Source: CAD feature listing. Evaluate the final solid. Frame: model axes, mm. Face numbers are marked on the shaded views. Give positions to 0.01 mm unless a question says otherwise; leave off trailing zeros. Order: outer loops, then holes, each group sorted by start corner. A loop starts at its lowest first (then second) coordinate and runs counter-clockwise, first axis right, second up.
1) First-contact query: P1, Ø6.5, axis at x = 42, y = 47.5, coming from the -Z side; P2, Ø10, axis at x = 44.5, z = 15.5, coming from the +Y side; P3, Ø2, axis at y = 30.5, z = 9, coming from the +X side; P4, Ø14.5, axis at y = 16, z = 44, coming from the -X side. Flat tips, straight axial feed; report the tip coordinate or a pass-through.
2) Section B-B, the plane z = 27. Return loops of the section in (x, y).
3) Material intervals for line 1 (X direction, y = 20, z = 32.5); line 2 (Z direction, x = 16.5, y = 19); line 3 (Y direction, x = 1.1, z = 44), sorted ascending.
4) Section A-A, the plane x = 12.5. Return loops of the section in (y, z).
5) Section C-C, the plane y = 9.5. Return loops of the section in (x, z).
6) Draft query along X for the marked faces 1, 2, 3 and 4. Return one class per face: released by +X, released by -X, zero draft, split by the parting line, or undercut.
7) Section D-D, the plane z = 7. Return loops of the section in (x, y).
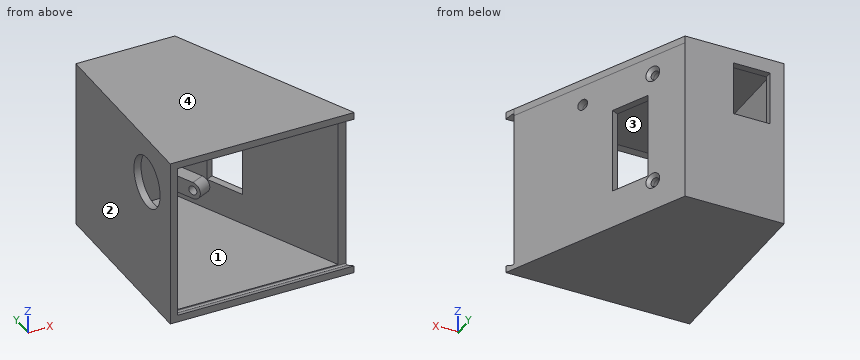
Autodesk Inventor part; units mm, degrees
ref_plane "Work Plane1" through (65, 0, 57.5) normal (1, 0, 0) x (0, 0, -1)
ref_plane "YZ Plane" through (0, 0, 0) normal (1, 0, 0) x (0, 1, 0)
ref_plane "XZ Plane" through (0, 0, 0) normal (0, 1, 0) x (-1, 0, 0)
sketch "Sketch1" plane through (0, 0, 0) normal (0, 0, 1) x (1, 0, 0)
  line L0 (0, 0) -> (0, 65)
  line L1 (0, 65) -> (35, 65)
  line L2 (35, 65) -> (65, 0)
  line L3 (65, 0) -> (0, 0)
  line L4 (35, 65) -> (19.5647, 57.876) construction
  line L5 (19.5647, 57.876) -> (40.0985, 13.386) construction
  line L6 (40.0985, 13.386) -> (55.5339, 20.51) construction
  line L7 (5, 65) -> (5, 39) construction
  line L8 (5, 39) -> (17.8, 39) construction
  line L9 (17.8, 39) -> (17.8, 65) construction
  line L10 (0, 23.6) -> (40, 23.6) construction
  line L11 (40, 23.6) -> (40, 6) construction
  line L12 (40, 6) -> (0, 6) construction
  line L13 (0, 26.5) -> (11, 26.5) construction
  line L14 (11, 26.5) -> (11, 23.6) construction
  line L15 (11, 6) -> (11, 3.1) construction
  line L16 (11, 3.1) -> (0, 3.1) construction
  dimension "d27" = 17
  dimension "d28" = 12.8
  dimension "d29" = 5
  dimension "d31" = 40
  dimension "d32" = 17.6
  dimension "d33" = 26
  dimension "d34" = 35
  dimension "d35" = 65
  dimension "d36" = 23.4
  dimension "d37" = 11
  dimension "d38" = 49
  dimension "d39" = 65
  dimension "d40" = 6
extrude "Extrusion1" add sketch "Sketch1" along normal blind 2.5
sketch "Sketch2" plane through (0, 0, 2.5) normal (0, 0, 1) x (1, 0, 0)
  line L0 (0, 65) -> (0, 0)
  line L1 (0, 0) -> (65, 0)
  line L2 (65, 0) -> (35, 65)
  line L3 (35, 65) -> (0, 65)
  line L4 (2.5, 2.5) -> (2.5, 62.5)
  line L5 (2.5, 62.5) -> (33.4004, 62.5)
  line L6 (33.4004, 62.5) -> (61.0927, 2.5)
  line L7 (61.0927, 2.5) -> (2.5, 2.5)
  line L8 (2.5, 2.5) -> (2.5, 0)
  line L9 (60.862, 3) -> (63.6154, 3)
  dimension "d2" = 2.5
  dimension "d3" = 3
extrude "Extrusion2" add sketch "Sketch2" along normal blind 55 contours L3 L2 L9 L6 L5 L4 L8 L1 L0
sketch "Sketch3" plane through (0, 0, 57.5) normal (0, 0, 1) x (1, 0, 0)
  line L0 (0, 65) -> (0, 0)
  line L1 (0, 0) -> (2.5, 0)
  line L2 (2.5, 0) -> (2.5, 62.5)
  line L3 (2.5, 62.5) -> (33.4004, 62.5)
  line L4 (33.4004, 62.5) -> (60.862, 3)
  line L5 (60.862, 3) -> (63.6154, 3)
  line L6 (63.6154, 3) -> (35, 65)
  line L7 (35, 65) -> (0, 65)
  line L8 (63.6154, 3) -> (65, 0)
  line L9 (65, 0) -> (2.5, 0)
extrude "Extrusion3" add sketch "Sketch3" along normal blind 2.5
sketch "Sketch4" plane through (0, 65, 0) normal (0, 1, 0) x (1, 0, 0)
  line L0 (5, -36) -> (18, -36)
  line L1 (18, -36) -> (18, -55)
  line L2 (18, -55) -> (5, -55)
  line L3 (5, -55) -> (5, -36)
  line L4 (0, 0) -> (0, -60)
  line L5 (35, -60) -> (0, -60)
  line L6 (4.1, -35.1) -> (18.9, -35.1) construction
  line L7 (18.9, -35.1) -> (18.9, -55.9) construction
  line L8 (18.9, -55.9) -> (4.1, -55.9) construction
  line L9 (4.1, -55.9) -> (4.1, -35.1) construction
  line L10 (5, -45.5) -> (4.1, -45.5) construction
  line L11 (18, -45.5) -> (18.9, -45.5) construction
  line L12 (11.5, -36) -> (11.5, -35.1) construction
  line L13 (11.5, -55) -> (11.5, -55.9) construction
  dimension "d41" = 13
  dimension "d42" = 19
  dimension "d43" = 14.8
  dimension "d44" = 20.8
  dimension "d45" = 5
  dimension "d46" = 5
extrude "Extrusion4" cut sketch "Sketch4" against normal through all
sketch "Sketch5" plane through (35, 65, 60) normal (0.9079594, 0.4190582, 0) x (0, 0, -1)
  line L0 (16.32, -14.8) -> (46.52, -14.8)
  line L1 (46.52, -14.8) -> (46.52, -29)
  line L2 (46.52, -29) -> (16.32, -29)
  line L3 (16.32, -29) -> (16.32, -14.8)
  circle A0 centre (9.42, -40.9) radius 1.95
  line L4 (60, -71.5891) -> (57.5, -71.5891)
  circle A1 centre (49.02, -12.9) radius 1.6
  circle A2 centre (9.02, -12.9) radius 1.6
  line L5 (9.02, -12.9) -> (49.02, -12.9) construction
  line L6 (60, 0) -> (0, 0)
  line L7 (3.5, -10) -> (53.82, -10) construction
  line L8 (53.82, -10) -> (53.82, -59.3) construction
  line L9 (53.82, -59.3) -> (3.5, -59.3) construction
  line L10 (3.5, -59.3) -> (3.5, -10) construction
  line L11 (0, -71.5891) -> (0, 0)
  point P0 (60, -44.3503)
  dimension "d17" = 40
  dimension "d18" = 3.2
  dimension "d19" = 30.2
  dimension "d20" = 14.2
  dimension "d47" = 2.5
  dimension "d48" = 1.9
  dimension "d49" = 28
  dimension "d50" = 39.6
  dimension "d51" = 50.32
  dimension "d52" = 4.8
  dimension "d53" = 49.3
  dimension "d54" = 2.9
  dimension "d55" = 10
  dimension "d72" = 3.5
  dimension "d73" = 3.9
extrude "Extrusion5" cut sketch "Sketch5" against normal up to next
sketch "Sketch6" plane through (0, 0, 0) normal (-1, 0, 0) x (0, 0, 1)
  circle A0 centre (44, 16) radius 9
  line L0 (0, 0) -> (60, 0)
  line L1 (60, 65) -> (60, 0)
  dimension "d56" = 18
  dimension "d57" = 7
  dimension "d58" = 7
extrude "Extrusion6" cut sketch "Sketch6" against normal up to next
ref_plane "Work Plane1" through (65, 0, 57.5) normal (1, 0, 0) x (0, 0, -1)
sketch "Sketch7" plane through (65, 0, 57.5) normal (1, 0, 0) x (0, 0, -1)
  line L0 (57.5, 65) -> (57.5, 0)
  line L1 (57.5, 65) -> (-2.5, 65)
  line L2 (-2.5, 0) -> (-2.5, 65)
  line L3 (0, 0) -> (-2.5, 0)
  line L4 (0, 0) -> (0, 3)
  line L5 (55, 3) -> (0, 3)
  line L6 (55, 0) -> (55, 3)
  line L7 (57.5, 0) -> (55, 0)
  line L8 (13.82, 38.6692) -> (13.82, 51.5622)
  line L9 (13.82, 51.5622) -> (44.02, 51.5622)
  line L10 (44.02, 51.5622) -> (44.02, 38.6692)
  line L11 (44.02, 38.6692) -> (13.82, 38.6692)
  ellipse E0 centre (6.92, 27.8645) end of major axis (4.97, 27.8645) minor radius 1.7705
  line L12 (0, 0) -> (-1, 3)
  line L13 (-1, 3) -> (0, 3)
  line L14 (55, 3) -> (56, 3)
  line L15 (56, 3) -> (55, 0)
  dimension "d59" = 1
extrude "Extrusion7" cut sketch "Sketch7" against normal up to surface (62.5 mm away) contours L6 L14 L15 | L12 L13 L4
fillet "Fillet1" radius 0.5 2 edges at (33.0577, 3, 58.5) (33.0577, 3, 1.5)
sketch "Sketch8" plane through (60.862, 3, 2.5) normal (-0.9079594, -0.4190582, 0) x (0, 0, 1)
  circle A0 centre (8.48, 54.2311) radius 1.6
  circle A1 centre (48.48, 54.2311) radius 1.6
  arc A2 (45.48, 54.2311) -> (51.48, 54.2311) centre (48.48, 54.2311) ccw
  line L0 (10.98, 52.3311) -> (41.18, 52.3311)
  line L1 (5.48, 54.2311) -> (5.48, 58.2311)
  line L2 (11.48, 58.2311) -> (11.48, 54.2311)
  line L3 (45.48, 54.2311) -> (45.48, 58.2311)
  line L4 (51.48, 58.2311) -> (51.48, 54.2311)
  line L5 (0, 65.5316) -> (55, 65.5316)
  arc A3 (5.48, 54.2311) -> (11.48, 54.2311) centre (8.48, 54.2311) ccw
  line L6 (5.48, 58.2311) -> (11.48, 58.2311)
  line L7 (45.48, 58.2311) -> (51.48, 58.2311)
  point P0 (-2.5, 22.7808)
  point P1 (6.9, 65.5316)
  point P2 (12.9, 65.5316)
  point P3 (46.9, 65.5316)
  point P4 (52.9, 65.5316)
  dimension "d60" = 3
  dimension "d61" = 4
extrude "Extrusion8" add sketch "Sketch8" along normal blind 4.8
sketch "Sketch12" plane through (36.4597, 55.8715, 53.98) normal (-0.4190582, 0.9079594, 0) x (0.9079594, 0.4190582, 0)
  line L0 (0, 6) -> (0, 0)
  line L1 (0, 6) -> (-4.8, 6)
  line L2 (-4.8, 0) -> (-4.8, 6)
  line L3 (0, 0) -> (-4.8, 0)
  line L4 (0, 46) -> (0, 40)
  line L5 (0, 46) -> (-4.8, 46)
  line L6 (-4.8, 40) -> (-4.8, 46)
  line L7 (0, 40) -> (-4.8, 40)
  point P0 (-56.5174, 53.98)
extrude "Extrusion11" add sketch "Sketch12" along normal up to next
sketch "Sketch13" plane through (35, 65, 60) normal (0.9079594, 0.4190582, 0) x (0, 0, -1)
  circle A0 centre (49.02, -12.9) radius 1.6
  circle A1 centre (9.02, -12.9) radius 1.6
  point P0 (60, -44.3503)
hole "Hole1" at (40.4059, 53.2873, 50.98) at (40.4059, 53.2873, 10.98) direction (-0.9079594, -0.4190582, 0) diameter 3 depth 20 tip angle 118 countersink diameter 5.5 countersink angle 90
sketch "Sketch14" plane through (60.862, 3, 2.5) normal (-0.9079594, -0.4190582, 0) x (0, 0, 1)
  line L0 (55, 65.5316) -> (55, 0)
  line L1 (10.98, 52.3311) -> (41.18, 52.3311)
  circle A0 centre (48.08, 26.2311) radius 1.95
  arc A1 (42.08, 26.2311) -> (54.08, 26.2311) centre (48.08, 26.2311) ccw
  line L2 (42.08, 26.2311) -> (42.08, 33.9811)
  line L3 (42.08, 33.9811) -> (54.08, 33.9811)
  line L4 (54.08, 33.9811) -> (54.08, 26.2311)
  arc A2 (54.08, 26.2311) -> (42.08, 26.2311) centre (48.08, 26.2311) ccw construction
  point P0 (-2.5, 22.7808)
  dimension "d71" = 12
  dimension "d80" = 1.75
extrude "Extrusion12" add sketch "Sketch14" along normal blind 1.75
chamfer "Chamfer1" distance 1.75 angle 45 1 edges at (45.033, 33.1201, 50.58)
properties part number "Caja temporizador"
From the geometry:
1. P1: stops at z = 0
1. P2: stops at y = 55.25
1. P3: stops at x = 51.38
1. P4: stops at x = 49.67
2. outline: (0, 0) - (2.5, 0) - (2.5, 62.5) - (33.4, 62.5) - (38.93, 50.51) - (41.2, 51.56) - (35, 65) - (0, 65) - close; (44.88, 37.62) - (60.86, 3) - (63.62, 3) - (47.15, 38.67) - close
3. line 1: x = 0 to 2.5, 53.02 to 55.77
3. line 2: z = 0 to 2.5, 57.5 to 60
3. line 3: y = 0 to 7, 25 to 65
4. outline: (0, 0) - (65, 0) - (65, 36) - (62.5, 36) - (62.5, 2.5) - (3, 2.5) - (3, 2.19) arc R0.5 cw to (2.34, 1.72) - (0, 2.5) - close; (0, 57.5) - (2.34, 58.28) arc R0.5 cw to (3, 57.81) - (3, 57.5) - (62.5, 57.5) - (62.5, 55) - (65, 55) - (65, 60) - (0, 60) - close
5. outline: (0, 0) - (60.62, 0) - (60.62, 60) - (0, 60) - (0, 50.22) - (2.5, 50.22) - (2.5, 57.5) - (57.86, 57.5) - (57.86, 2.5) - (2.5, 2.5) - (2.5, 37.78) - (0, 37.78) - close
6. face 1: undercut
6. face 2: released by -X
6. face 3: undercut
6. face 4: zero draft
7. outline: (0, 0) - (2.5, 0) - (2.5, 62.5) - (33.4, 62.5) - (60.86, 3) - (63.62, 3) - (35, 65) - (0, 65) - close
